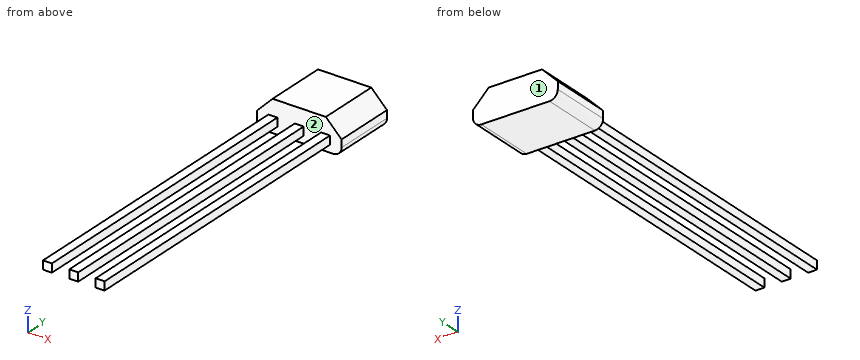
```python
from build123d import *

# Parameters (mm, degrees)
BOSS_EXTRUDE1_DEPTH = 3.02
SKETCH3_W           = 0.43
SKETCH3_H           = 14.99
BOSS_EXTRUDE2_DEPTH = 0.41


with BuildPart() as part:
    # Sketch2 → Boss-Extrude1 (new body)
    with BuildSketch(Plane(origin=(0, 0, 0), x_dir=(1, 0, 0), z_dir=(0, 1, 0))):
        with BuildLine():
            Line((-1.645, 0.76), (1.645, 0.76))
            ThreePointArc((1.645, 0.76), (1.927842712, 0.642842712), (2.045, 0.36))
            Line((2.045, 0.36), (2.045, 0))
            Line((2.045, 0), (1.285, -0.76))
            Line((1.285, -0.76), (-1.285, -0.76))
            Line((-1.285, -0.76), (-2.045, 0))
            Line((-2.045, 0), (-2.045, 0.36))
            ThreePointArc((-2.045, 0.36), (-1.927842712, 0.642842712), (-1.645, 0.76))
        make_face()
    extrude(amount=BOSS_EXTRUDE1_DEPTH)

    # Sketch3 → Boss-Extrude2 (add)
    with BuildSketch(Plane.XY):
        with Locations((0, -7.495)):
            Rectangle(SKETCH3_W, SKETCH3_H)
        with Locations((1.27, -7.495)):
            Rectangle(SKETCH3_W, SKETCH3_H)
        with Locations((-1.27, -7.495)):
            Rectangle(SKETCH3_W, SKETCH3_H)
    extrude(amount=-BOSS_EXTRUDE2_DEPTH)


solid = part.part
```
Read the model definition and answer for the solid it produces. Units are mm, in the model's axes. Face numbers are marked on the shaded views. Coordinates: 2 decimals unless noted, no trailing zeros. Write each loop counter-clockwise with the first axis right and the second up, starting at its lowest first coordinate (ties: lowest second). Pieces come first, ordered by that corner, then holes. Notation, with made-up numbers: (-5.5, -7) -> (39.5, -7) arc R25 ccw to (39.5, 10) -> close; hole circle Ø2 at (-12.75, -4.75). An arc over 180 degrees is marked (long way). Answer as a JSON object with one key per item and string values.
Q1. Flat-ended cylindrical pins translate along their axes: pin 1 Ø0.5 at (x, y) = (1, -8) entering from -Z; pin 2 Ø0.5 at (y, z) = (-4, -0.5) entering from +X (3 decimals); pin 3 Ø0.5 at (y, z) = (-10.5, 0) entering from -X (3 decimals). Find the tip coordinate at first contact, or state that the pin passes through.
The answers:
{"pin 1": "stops at z = -0.41", "pin 2": "stops at x = 1.485", "pin 3": "stops at x = -1.485"}
Q2. The part is cut by section C-C on z = 0.4. Give the vertices of the cut face in (x, y) (3 decimals).
The answers:
{"outline": "(-1.645, 0) -> (1.645, 0) -> (1.645, 3.02) -> (-1.645, 3.02) -> close"}
Q3. The part is cut by section B-B on x = 0.4. Give the vertices of the cut face in (y, z).
The answers:
{"outline": "(0, -0.76) -> (3.02, -0.76) -> (3.02, 0.76) -> (0, 0.76) -> close"}
Q4. Consider line 1 (X direction, y = -2.25, z = -0.1) (3 decimals); line 2 (Y direction, x = 1.1, z = 0.6); line 3 (Z direction, x = 0.05, y = -7). Determine where each line is inside the solid, lowest interval first. Write a range as [from, to].
The answers:
{"line 1": "x = [-1.485, -1.055], [-0.215, 0.215], [1.055, 1.485]", "line 2": "y = [0, 3.02]", "line 3": "z = [-0.41, 0]"}
Q5. The part is cut by section A-A on y = -4.75. Give the vertices of the cut face in (x, z) (3 decimals), then the cut area to 3 significant figures.
The answers:
{"outline": "(-1.485, -0.41) -> (-1.055, -0.41) -> (-1.055, 0) -> (-1.485, 0) -> close; (-0.215, -0.41) -> (0.215, -0.41) -> (0.215, 0) -> (-0.215, 0) -> close; (1.055, -0.41) -> (1.485, -0.41) -> (1.485, 0) -> (1.055, 0) -> close", "area": "0.529 mm2"}
Q6. Determine the mould class of the marked faces 1 and 2 for opening direction X: pulls with the +X half, pulls with the -X half, needs draft (parallel to the pull), parting line crosses it, or undercut.
The answers:
{"face 1": "needs draft", "face 2": "undercut"}
